```python
from build123d import *

# Parameters (mm, degrees)
SKETCH_1_R             = 3.96875
SKETCH_1_R_2           = 3.571875
BOSS_EXTRUDE1_DEPTH    = 6.35
FILLET1_START          = -1
FILLET1_DEPTH          = 8
FILLET1_2_DEPTH        = 6.35
F_10_24_TAPPED_HOLE1_D = 3.7973


with BuildPart() as part:
    # Sketch 1 → Boss-Extrude1 (new body)
    with BuildSketch(Plane.XY):
        with BuildLine():
            Line((-11.214382662, 4.081701485), (-10.004213371, 7.406614284))
            Line((-10.004213371, 7.406614284), (-1.650345972, 4.36605521))
            Line((-1.650345972, 4.36605521), (20.067934728, 64.036536047))
            Line((20.067934728, 64.036536047), (70.64649272, 45.627444911))
            Line((70.64649272, 45.627444911), (55.009330616, 2.664698708))
            Line((55.009330616, 2.664698708), (63.363198014, -0.375860367))
            Line((63.363198014, -0.375860367), (63.5, 0))
            Line((63.5, 0), (62.014382214, -4.081701322))
            ThreePointArc((62.014382214, -4.081701322), (57.645116691, -9.775839758), (50.8, -11.934096761))
            Line((50.8, -11.934096761), (0, -11.934096761))
            ThreePointArc((0, -11.934096761), (-9.775839758, -6.845116691), (-11.214382662, 4.081701485))
        make_face()
        with Locations((50.8, 0)):
            Circle(SKETCH_1_R, mode=Mode.SUBTRACT)
        with Locations((54.351671245, 16.419125005)):
            Circle(SKETCH_1_R_2, mode=Mode.SUBTRACT)
        with Locations((13.775744275, 31.187555882)):
            Circle(SKETCH_1_R_2, mode=Mode.SUBTRACT)
        with Locations((22.463055915, 55.05574845)):
            Circle(SKETCH_1_R_2, mode=Mode.SUBTRACT)
        with Locations((63.038982885, 40.287317573)):
            Circle(SKETCH_1_R_2, mode=Mode.SUBTRACT)
        with BuildLine():
            Line((29.996461326, 29.338214557), (40.737147877, 25.428924031))
            ThreePointArc((40.737147877, 25.428924031), (43.014279885, 20.545598338), (38.130954193, 18.26846633))
            Line((38.130954193, 18.26846633), (27.390267642, 22.177756856))
            ThreePointArc((27.390267642, 22.177756856), (25.113135634, 27.061082549), (29.996461326, 29.338214557))
        make_face(mode=Mode.SUBTRACT)
        with BuildLine():
            Line((36.077579283, 46.045949424), (46.818265834, 42.136658898))
            ThreePointArc((46.818265834, 42.136658898), (51.701591526, 44.413790906), (49.424459518, 49.297116599))
            Line((49.424459518, 49.297116599), (38.683772967, 53.206407125))
            ThreePointArc((38.683772967, 53.206407125), (33.800447275, 50.929275117), (36.077579283, 46.045949424))
        make_face(mode=Mode.SUBTRACT)
        Polygon((14.530404991, 14.694812411), (9.752383236, 1.567306626), (38.394214039, -8.85746811), (43.172235793, 4.270037674), align=None, mode=Mode.SUBTRACT)
        Polygon((21.809316491, 45.833149672), (57.611604993, 32.802181251), (55.005411309, 25.641723551), (19.203122807, 38.672691971), align=None, mode=Mode.SUBTRACT)
    extrude(amount=BOSS_EXTRUDE1_DEPTH)

    # Fillet1: read off the stored shape, not the designer's step
    # Fillet1 outline → Fillet1 (cut)
    with BuildSketch(Plane.XY.offset(FILLET1_START)):
        with BuildLine():
            Line((63.363198014, -0.375860367), (60.976378758, 0.492870798))
            ThreePointArc((60.976378758, 0.492870798), (62.409669373, -0.820498074), (62.49446685, -2.762679623))
            Line((62.49446685, -2.762679623), (63.363198014, -0.375860367))
        make_face()
        with BuildLine():
            ThreePointArc((-10.872944535, 5.019795027), (-9.559575663, 6.453085642), (-7.617394114, 6.53788312))
            Line((-7.617394114, 6.53788312), (-10.004213371, 7.406614284))
            Line((-10.004213371, 7.406614284), (-10.872944535, 5.019795027))
        make_face()
        with BuildLine():
            ThreePointArc((19.1992035, 61.649716814), (20.512572411, 63.083007394), (22.454753962, 63.167804819))
            Line((22.454753962, 63.167804819), (20.067934728, 64.036536047))
            Line((20.067934728, 64.036536047), (19.1992035, 61.649716814))
        make_face()
        with BuildLine():
            ThreePointArc((68.259673487, 46.496176139), (69.692964066, 45.182807228), (69.777761492, 43.240625677))
            Line((69.777761492, 43.240625677), (70.64649272, 45.627444911))
            Line((70.64649272, 45.627444911), (68.259673487, 46.496176139))
        make_face()
    extrude(amount=FILLET1_DEPTH, mode=Mode.SUBTRACT)

    # Fillet1 2 outline → Fillet1 2 (add)
    with BuildSketch(Plane.XY):
        with BuildLine():
            Line((-1.650345972, 4.36605521), (-0.781614768, 6.752874379))
            ThreePointArc((-0.781614768, 6.752874379), (-2.094983647, 5.319583814), (-4.037165165, 5.23478635))
            Line((-4.037165165, 5.23478635), (-1.650345972, 4.36605521))
        make_face()
        with BuildLine():
            Line((55.009330616, 2.664698708), (57.396149936, 1.79596752))
            ThreePointArc((57.396149936, 1.79596752), (55.962859307, 3.109336423), (55.878061867, 5.051518005))
            Line((55.878061867, 5.051518005), (55.009330616, 2.664698708))
        make_face()
        with BuildLine():
            ThreePointArc((40.785416559, 5.138768902), (42.218707139, 3.825399992), (42.303504565, 1.883218441))
            Line((42.303504565, 1.883218441), (43.172235793, 4.270037674))
            Line((43.172235793, 4.270037674), (40.785416559, 5.138768902))
        make_face()
        with BuildLine():
            Line((38.394214039, -8.85746811), (39.262945267, -6.470648877))
            ThreePointArc((39.262945267, -6.470648877), (37.949576356, -7.903939456), (36.007394805, -7.988736882))
            Line((36.007394805, -7.988736882), (38.394214039, -8.85746811))
        make_face()
        with BuildLine():
            ThreePointArc((13.661673763, 12.307993177), (14.975042673, 13.741283757), (16.917224224, 13.826081183))
            Line((16.917224224, 13.826081183), (14.530404991, 14.694812411))
            Line((14.530404991, 14.694812411), (13.661673763, 12.307993177))
        make_face()
        with BuildLine():
            Line((9.752383236, 1.567306626), (12.13920247, 0.698575398))
            ThreePointArc((12.13920247, 0.698575398), (10.70591189, 2.011944309), (10.621114464, 3.95412586))
            Line((10.621114464, 3.95412586), (9.752383236, 1.567306626))
        make_face()
        with BuildLine():
            ThreePointArc((55.874142537, 28.028542784), (54.560773627, 26.595252204), (52.618592076, 26.510454779))
            Line((52.618592076, 26.510454779), (55.005411309, 25.641723551))
            Line((55.005411309, 25.641723551), (55.874142537, 28.028542784))
        make_face()
        with BuildLine():
            Line((19.203122807, 38.672691971), (21.58994204, 37.803960743))
            ThreePointArc((21.58994204, 37.803960743), (20.15665146, 39.117329653), (20.071854035, 41.059511204))
            Line((20.071854035, 41.059511204), (19.203122807, 38.672691971))
        make_face()
        with BuildLine():
            ThreePointArc((55.22478576, 33.670912479), (56.65807634, 32.357543569), (56.742873765, 30.415362018))
            Line((56.742873765, 30.415362018), (57.611604993, 32.802181251))
            Line((57.611604993, 32.802181251), (55.22478576, 33.670912479))
        make_face()
        with BuildLine():
            Line((21.809316491, 45.833149672), (20.940585263, 43.446330438))
            ThreePointArc((20.940585263, 43.446330438), (22.253954173, 44.879621018), (24.196135724, 44.964418443))
            Line((24.196135724, 44.964418443), (21.809316491, 45.833149672))
        make_face()
    extrude(amount=FILLET1_2_DEPTH)

    # 10-24 Tapped Hole1 (through all)
    with Locations(Plane.XY.offset(6.35)):
        with Locations((0, 0)):
            Hole(F_10_24_TAPPED_HOLE1_D / 2)


solid = part.part
```
Geometry: final body of the model. Coordinates: model frame, mm. A direction names the side the tool comes from. Round coordinates to 2 decimals unless told otherwise and drop trailing zeros. Write item = value, one per line. Start each with the question number.
Q1. Ray query, line 1 (Y direction, x = 24, z = 4); line 2 (Y direction, x = 33, z = 2); line 3 (Y direction, x = 35, z = 2.25). Return the intervals inside material, ascending. Write a range as from..to.
Q2. Access query for faces 1 (the flat face through (59.161, 1.154, 3.131)), 2 (the flat face through (26, -11.934, 3)), 3 (the flat face through (35.29, 27.41, 3.13)). Directions: +Z, -Z, +X, -X, +Y, -Y. A direction counts if a zero-diameter tool reaches every point of the face in a straight line with its end or side. Return the directions, or none.
Q3. Pull-direction query (Y, two-part tool) for faces 4 (the cylindrical face through (-2.07, 5.33, 3.13)), 5 (the cylindrical face through (-1.8, 0.6, 3.1)), 6 (the flat face through (62.925, 24.413, 3.131)), 7 (the cylindrical face through (-9.68, -6.98, 3.13)); classes: +Y half, -Y half, draft (parallel to the pull), parting line (faces both ways), or undercut.
Q4. Pin query (flat end, axial travel): pin 1 (3 mm diameter, centred on x = 57, z = 4.5, fed in from -Y); pin 2 (5.5 mm diameter, centred on x = 22.46, y = 55.06, fed in from -Z). Return the tip coordinate at first contact, or that it passes through.
Outcome:
q1.line_1 = -11.93..-3.62, 11.25..36.93, 45.03..51.83, 58.28..62.61
q1.line_2 = -11.93..-6.89, 7.97..20.14, 28.25..33.65, 41.76..59.33
q1.line_3 = -11.93..-7.62, 7.24..19.41, 27.52..32.92, 41.03..46.65, 52.6..58.6
q2.face_1 = +Z, -Z, +X
q2.face_2 = +Z, -Z, +X, -X, -Y
q2.face_3 = +Z, -Z
q3.face_4 = +Y half
q3.face_5 = undercut
q3.face_6 = undercut
q3.face_7 = parting line
q4.pin_1 = -10.97
q4.pin_2 = through
